Autodesk Inventor part; units mm, degrees
ref_plane "Work Plane1" through (-20.8033, -6.3, -5.9) normal (0, 0, 1) x (1, 0, 0)
ref_plane "YZ Plane" through (0, 0, 0) normal (1, 0, 0) x (0, 1, 0)
ref_plane "XZ Plane" through (0, 0, 0) normal (0, 1, 0) x (-1, 0, 0)
sketch "Sketch1" plane through (0, 0, 0) normal (0, 0, 1) x (1, 0, 0)
  line L0 (0.8467, -0.7217) -> (0.8467, 0.7217) construction
  line L1 (0.8467, 0.7217) -> (2.0967, 1.4434) construction
  line L2 (2.0967, 1.4434) -> (3.3467, 0.7217) construction
  line L3 (3.3467, 0.7217) -> (3.3467, -0.7217) construction
  line L4 (3.3467, -0.7217) -> (2.0967, -1.4434) construction
  line L5 (2.0967, -1.4434) -> (0.8467, -0.7217) construction
  circle A0 centre (2.0967, 0) radius 2.45 construction
  line L6 (4.8467, -1.5877) -> (3.4717, -2.3816) construction
  line L7 (15.0967, 3) -> (15.0967, -3) construction
  line L8 (-10.9033, 3) -> (-10.9033, -3) construction
  line L9 (-0.6533, 0) -> (-0.6533, 1.5877) construction
  circle A1 centre (2.0967, 0) radius 5
  circle A2 centre (2.0967, 0) radius 1.7
  line L10 (-10.9033, -3) -> (15.0967, -3)
  line L11 (-10.9033, 3) -> (15.0967, 3)
  circle A3 centre (2.0967, 0) radius 3.5
  circle A4 centre (2.0967, 0) radius 6.5
  point P0 (0.4719, -0.5)
  point P1 (3.7215, -0.5)
  dimension "d10" = 7
  dimension "d13" = 13
ref_plane "Work Plane1" through (-20.8033, -6.3, -5.9) normal (0, 0, 1) x (1, 0, 0)
extrude "Extrusion1" add sketch "Sketch1" against normal blind 1 contours A1 L10 A3 L11 | A1 L11 A4 L10 | L11 A3 A1 | A1 L11 A4 | L10 A4 A1 | A1 L10 A3 | L11 A3 L10 A1 | A1 L10 A4 L11 | A3 L10 L11 | L11 A3 | A3 L10 | A2
sketch "Sketch2" plane through (2.0967, 0, 0) normal (0, 0, 1) x (1, 0, 0)
  line L0 (-2, 1.5) -> (2, 1.5) construction
  arc A0 (2.5, 0) -> (2, 1.5) centre (0, 0) ccw construction
  arc A1 (-2, 1.5) -> (-2.5, 0) centre (0, 0) ccw construction
  line L1 (2, -1.5) -> (-2, -1.5) construction
  arc A2 (-2.5, 0) -> (2.5, 0) centre (0, 0) ccw construction
  line L2 (2.0248, 1.55) -> (-2.0248, 1.55) construction
  arc A3 (-2.0248, 1.55) -> (-2.55, 0) centre (0, 0) ccw construction
  arc A4 (-2.55, 0) -> (2.55, 0) centre (0, 0) ccw construction
  arc A5 (2.55, 0) -> (2.0248, 1.55) centre (0, 0) ccw construction
  line L3 (-2.0248, 1.55) -> (2.0248, 1.55) construction
  line L4 (-2.0248, 1.55) -> (2.0248, 1.55)
  line L5 (-2.0248, -1.55) -> (2.0248, -1.55)
  arc A6 (-2.0248, 1.55) -> (-2.0248, -1.55) centre (0, 0) ccw
  arc A7 (2.0248, -1.55) -> (2.0248, 1.55) centre (0, 0) ccw
  circle A8 centre (0, 0) radius 6.5
  circle A9 centre (0, 0) radius 2.5
  point P0 (-2.0967, 0)
  point P1 (-1.9615, 1.55)
  point P2 (1.9615, 1.55)
  point P3 (1.9615, -1.55)
  point P4 (-1.9615, -1.55)
  dimension "d11" = 3.1
  dimension "d12" = 2.55
extrude "Extrusion2" add sketch "Sketch2" along normal blind 10
sketch "Sketch4" plane through (0.0718, -1.55, 0) normal (0, 1, 0) x (1, 0, 0)
  line L0 (0, -8.8) -> (4.0497, -8.8)
  line L1 (-4.4752, -10) -> (8.5248, -10)
  line L2 (8.5248, 1) -> (-4.4752, 1)
  line L3 (0, 0) -> (0.0633, 0)
  circle A0 centre (2.0248, -2.0248) radius 2.0248
  line L4 (3.9864, 0) -> (4.0497, 0)
  line L5 (3.9864, 0) -> (3.9864, -10)
  line L6 (4.0497, -10) -> (3.9864, -10)
  line L7 (4.0497, 0) -> (4.0497, -10)
  line L8 (0, 0) -> (0, -10)
  line L9 (0.0633, -10) -> (0, -10)
  line L10 (0.0633, 0) -> (0.0633, -10)
  point P0 (-0.0718, 0)
hole "Hole1" at (2.0967, -1.55, 2.0248) direction (0, -1, 0) diameter 2.5 end through all both
sketch "Skizze5" plane through (2.0967, 0, -1) normal (0, 0, -1) x (-1, 0, 0)
  circle A0 centre (0, 0) radius 6.5
  line L0 (22.5, -4.5) -> (-22.5, -4.5)
  line L1 (-22.5, -4.5) -> (-22.5, 4.5)
  line L2 (-22.5, 4.5) -> (22.5, 4.5)
  line L3 (22.5, 4.5) -> (22.5, -4.5)
  line L4 (22.5, -4.5) -> (-22.5, 4.5) construction
  line L5 (-22.5, -4.5) -> (22.5, 4.5) construction
  circle A1 centre (0, 0) radius 2.5
  line L6 (12, 4.5) -> (12, -4.5)
  point P0 (2.0967, 0)
  dimension "d28" = 45
  dimension "d34" = 9
  dimension "d35" = 12
extrude "Extrusion4" add sketch "Skizze5" along normal blind 6 contours A0 L0 L2 | A0 L2 L6 L0 | A0 L0 L1 L2
properties part number "55_spiralxy_motormount_NEMA_MGN7"
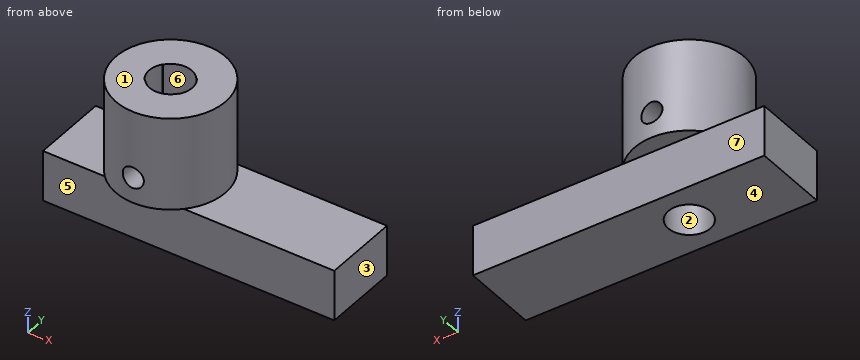
The listing builds one solid part. Answer for the finished solid, in the listing's coordinates (mm). Face numbers are marked on the shaded views. A direction names the side the tool comes from. Coordinates: 2 decimals unless noted, no trailing zeros. Write each loop counter-clockwise with the first axis right and the second up, starting at its lowest first coordinate (ties: lowest second). Pieces come first, ordered by that corner, then holes. Notation, with made-up numbers: M -12,55.25 L 32,55.25 A23 cw 32,78.25 Z; hole C -27.5,-10.75 d8. An arc over 180 degrees is marked long. Use a Markdown table: item, result. Add a question column.
1. Section A-A (z = -4.5) is taken. Give the vertices of the cut face in (x, y).
2. Which of the six approach directions +Z, -Z, +X, -X, +Y, -Y give full straight-line access (tool end or side, diameter ignored) to the marked faces 4, 5, 6 and 7?
3. Straight lines are drawn through the part: line 1 along Z through (x, y) = (19, 1.75); line 2 along Y through (x, z) = (2, -1.5); line 3 along X through (y, z) = (1.5, 2.5). For each, find the intervals that lie inside material, in ascending order. Write a range as [from, to].
4. Section C-C (y = 3) is taken. Give the vertices of the cut face in (x, z), plus the area to 3 significant figures.
5. Section B-B (y = 0) is taken. Give the vertices of the cut face in (x, z).
6. Given P1, Ø2.5, axis at x = 1, y = 0, coming from the +Z side; P2, Ø3, axis at y = 2, z = 2.5, coming from the +X side; P3, Ø4, axis at x = 13.5, y = 4, coming from the +Z side, each flat-ended and moving along its own axis, determine where each tip first touches the part or whether it passes through.
7. For a pull along X with two mould halves and no side action, classify the marked faces 1, 2 and 3 as +X half, -X half, draft (parallel to the pull), parting line (faces both ways), or undercut.
8. Section D-D (x = 12.5) is taken. Give the vertices of the cut face in (y, z), plus the area to 3 significant figures.
Data:
| question | item | result |
|---|---|---|
| 1 | outline | M -9.9,-4.5 L 24.6,-4.5 L 24.6,4.5 L -9.9,4.5 Z; hole C 2.1,0 d5 |
| 2 | face 4 | -Z, +X, -X, +Y, -Y |
| 2 | face 5 | -Z, +X, -X, -Y |
| 2 | face 6 | +Z |
| 2 | face 7 | -Z, +X, -X, +Y |
| 3 | line 1 | z = [-7, -1] |
| 3 | line 2 | y = [-4.5, -2.5], [2.5, 4.5] |
| 3 | line 3 | x = [-4.23, 0.03], [4.16, 8.42] |
| 4 | outline | M -9.9,-7 L 24.6,-7 L 24.6,-1 L 7.86,-1 L 7.86,10 L -3.67,10 L -3.67,-1 L -9.9,-1 Z; hole C 2.1,2.02 d2.5 |
| 4 | area | 329 mm2 |
| 5 | outline | M -9.9,-7 L -0.4,-7 L -0.4,-1 L 4.6,-1 L 4.6,-7 L 24.6,-7 L 24.6,-1 L 8.6,-1 L 8.6,10 L 4.65,10 L 4.65,0 L -0.45,0 L -0.45,10 L -4.4,10 L -4.4,-1 L -9.9,-1 Z |
| 6 | P1 | stops at z = 0 |
| 6 | P2 | stops at x = 8.58 |
| 6 | P3 | stops at z = -1 |
| 7 | face 1 | draft |
| 7 | face 2 | undercut |
| 7 | face 3 | +X half |
| 8 | outline | M -4.5,-7 L 4.5,-7 L 4.5,-1 L -4.5,-1 Z |
| 8 | area | 54.0 mm2 |
